```python
from build123d import *

# Parameters (mm, degrees)
SKETCH1_W               = 80
SKETCH1_H               = 35
BOSS_EXTRUDE1_DEPTH     = 35
CUT_EXTRUDE1_DEPTH      = 45
SKETCH3_W               = 35
SKETCH3_H               = 35
BOSS_EXTRUDE2_DEPTH     = 10
SKETCH4_W               = 15
SKETCH4_H               = 15
CUT_EXTRUDE2_DEPTH      = 1
CUT_EXTRUDE2_DEPTH_BACK = 36
SKETCH5_R               = 5
CUT_EXTRUDE3_DEPTH      = 10
SKETCH6_W               = 25
SKETCH6_H               = 5
CUT_EXTRUDE4_DEPTH      = 36
SKETCH7_R               = 7.5
CUT_EXTRUDE5_DEPTH      = 36


with BuildPart() as part:
    # Sketch1 → Boss-Extrude1 (new body)
    with BuildSketch(Plane(origin=(0, 0, 0), x_dir=(1, 0, 0), z_dir=(0, 1, 0))):
        with Locations((40, 17.5)):
            Rectangle(SKETCH1_W, SKETCH1_H)
    extrude(amount=BOSS_EXTRUDE1_DEPTH)

    # Sketch2 → Cut-Extrude1 (cut)
    with BuildSketch(Plane(origin=(80, 0, 0), x_dir=(0, 0, -1), z_dir=(1, 0, 0))):
        Polygon((35, 35), (35, 25), (0, 10), (0, 35), align=None)
    extrude(amount=-CUT_EXTRUDE1_DEPTH, mode=Mode.SUBTRACT)

    # Sketch3 → Boss-Extrude2 (add)
    with BuildSketch(Plane(origin=(80, 0, 0), x_dir=(0, 0, -1), z_dir=(1, 0, 0))):
        with Locations((17.5, 17.5)):
            Rectangle(SKETCH3_W, SKETCH3_H)
    extrude(amount=-BOSS_EXTRUDE2_DEPTH)

    # Sketch4 → Cut-Extrude2 (cut, two sides)
    with BuildSketch(Plane(origin=(0, 0, 0), x_dir=(-1, 0, 0), z_dir=(0, -1, 0))) as cut_extrude2_sk:
        with Locations((-42.5, 7.5)):
            Rectangle(SKETCH4_W, SKETCH4_H)
    extrude(amount=CUT_EXTRUDE2_DEPTH, mode=Mode.SUBTRACT)
    extrude(cut_extrude2_sk.sketch, amount=-CUT_EXTRUDE2_DEPTH_BACK, mode=Mode.SUBTRACT)

    # Sketch5 → Cut-Extrude3 (cut)
    with BuildSketch(Plane(origin=(80, 0, 0), x_dir=(0, 0, -1), z_dir=(1, 0, 0))):
        with Locations((10, 25)):
            Circle(SKETCH5_R)
    extrude(amount=-CUT_EXTRUDE3_DEPTH, mode=Mode.SUBTRACT)

    # Sketch6 → Cut-Extrude4 (cut, through all)
    with BuildSketch(Plane.XY):
        with Locations((17.5, 2.5)):
            Rectangle(SKETCH6_W, SKETCH6_H)
    extrude(amount=-CUT_EXTRUDE4_DEPTH, mode=Mode.SUBTRACT)

    # Sketch7 → Cut-Extrude5 (cut, through all)
    with BuildSketch(Plane(origin=(0, 35, 0), x_dir=(1, 0, 0), z_dir=(0, 1, 0))):
        with Locations((17.5, 17.5)):
            Circle(SKETCH7_R)
    extrude(amount=-CUT_EXTRUDE5_DEPTH, mode=Mode.SUBTRACT)


solid = part.part
```
Geometry check sheet. Reference: the model listing, model coordinates, mm. A direction names the side the tool comes from. Coordinates: 2 decimals unless noted, no trailing zeros. Order: outer loops, then holes, each group sorted by start corner. A loop starts at its lowest first (then second) coordinate and runs counter-clockwise, first axis right, second up. Notation, with made-up numbers: (37.25, 7.25) - (45.25, 7.25) arc R20 ccw to (45.25, 40.25) - close; hole circle Ø7 at (16, -5.5). An arc over 180 degrees is marked (long way). Use one line per item in the form item = value.
1. Gauge pin test, flat ends, axial feed: pin 1 (1.5 mm diameter, centred on x = 21, z = -4.5, fed in from -Y); pin 2 (4.5 mm diameter, centred on x = 44, y = 11, fed in from +Z); pin 3 (9 mm diameter, centred on x = 17.5, z = -17.5, fed in from +Y); pin 4 (10 mm diameter, centred on x = 59, z = -21, fed in from +Y). Record the tip position at first contact, or that the pin passes through.
Here are the results:
pin_1 = 5
pin_2 = -15
pin_3 = through
pin_4 = 21.14
2. Draft check along Z on faces 6 (the face through (39, 17, -35)), 7 (the face through (75.07, 20.564, -12.307)), 8 (the face through (12, 20.2, -22.6)), 9 (the face through (5, 2, -17)). Enter one of: pulls with the +Z half, pulls with the -Z half, needs draft (parallel to the pull), parting line crosses it, or undercut.
Here are the results:
face_6 = pulls with the -Z half
face_7 = undercut
face_8 = undercut
face_9 = needs draft
3. Scan lines: line 1 (X direction, y = 19, z = -17); line 2 (Y direction, x = 73.5, z = -10); line 3 (X direction, y = 23.5, z = -25.5). Record each from-to range of solid material in increasing order.
Here are the results:
line_1 = 0 to 10.02, 24.98 to 35, 70 to 80
line_2 = 0 to 20, 30 to 35
line_3 = 0 to 35, 70 to 80
4. Section check C-C (z = -17.5). Record the boundary of the cut face in (x, y).
Here are the results:
outline = (0, 0) - (5, 0) - (5, 5) - (10, 5) - (10, 35) - (0, 35) - close; (25, 5) - (30, 5) - (30, 0) - (80, 0) - (80, 35) - (70, 35) - (70, 17.5) - (35, 17.5) - (35, 35) - (25, 35) - close
5. Section check B-B (x = 17.5). Record the boundary of the cut face in (y, z).
Here are the results:
outline = (5, -35) - (35, -35) - (35, -25) - (5, -25) - close; (5, -10) - (35, -10) - (35, 0) - (5, 0) - close
6. Access from +Z, -Z, +X, -X, +Y, -Y to the whole of each face (thin tool, end or side, straight path). Record for faces 1 (the face through (43, 8, -15)), 2 (the face through (80, 17, -17)), 3 (the face through (70, 25, -17)), 4 (the face through (2, 0, -18)), 5 (the face through (17, 5, -9)).
Here are the results:
face_1 = +Z, +Y, -Y
face_2 = +Z, -Z, +X, +Y, -Y
face_3 = +Z, +Y
face_4 = +Z, -Z, +X, -X, -Y
face_5 = +Z, -Z, -Y
7. Section check A-A (y = 22). Record the boundary of the cut face in (x, z).
Here are the results:
outline = (0, -35) - (80, -35) - (80, -14) - (70, -14) - (70, -28) - (35, -28) - (35, 0) - (0, 0) - close; (70, -6) - (80, -6) - (80, 0) - (70, 0) - close; hole circle Ø15 at (17.5, -17.5)
8. Section check D-D (x = 72.5). Record the boundary of the cut face in (y, z), then the cut area to 3 significant figures.
Here are the results:
outline = (0, -35) - (35, -35) - (35, 0) - (0, 0) - close; hole circle Ø10 at (25, -10)
area = 1,150 mm²
